Could you check a few things on this model? Use its own coordinates, in mm. Round coordinates to 2 decimals unless told otherwise and drop trailing zeros. Loops run counter-clockwise (first coordinate to the right, second up) from the corner with the lowest first, then second, coordinate; pieces in that order, holes last. Notation, with made-up numbers: M 72,27.5 L 80,27.5 A18 cw 80,33.5 Z; hole C -4,79 d3. An arc over 180 degrees is marked long. Answer in a Markdown table with one row per item.
Autodesk Inventor part; units mm, degrees
ref_plane "YZ Plane" through (0, 0, 0) normal (1, 0, 0) x (0, 1, 0)
ref_plane "XZ Plane" through (0, 0, 0) normal (0, 1, 0) x (-1, 0, 0)
ref_plane "XY Plane" through (0, 0, 0) normal (0, 0, 1) x (1, 0, 0)
ref_plane "Work Plane1" through (-228.0882, -76.2, -228.6) normal (0, 1, 0) x (-1, 0, 0)
sketch "Sketch2" plane through (-228.0882, -76.2, -228.6) normal (0, 1, 0) x (-1, 0, 0)
  circle A0 centre (-228.6, 228.6) radius 227.5764 construction
  circle A1 centre (-228.6, 228.6) radius 228.6 construction
  arc A2 (-228.6, 1.0236) -> (-25.4, 126.1267) centre (-228.6, 228.6) ccw construction
  arc A3 (-228.6, 0) -> (-25.4, 123.8731) centre (-228.6, 228.6) ccw construction
  line L0 (-228.6, 0) -> (-25.4, 0)
  arc A4 (-228.6, 1.0236) -> (-25.4, 126.1267) centre (-228.6, 228.6) ccw
  line L1 (-228.6, 228.6) -> (-25.4, 126.1267) construction
  line L2 (-228.6, 228.6) -> (-228.6, 1.0236) construction
  line L3 (-25.4, 126.1267) -> (-25.4, 0)
  line L4 (-228.6, 0) -> (-228.6, 1.0236)
  line L5 (-228.6, 0) -> (-228.6, 1.0236)
  line L6 (-25.4, 123.8731) -> (-25.4, 126.1267)
  point P0 (-228.0882, 228.6)
  point P1 (-1.0236, 228.6)
  point P2 (0, 228.6)
  point P3 (-228.6, 228.6)
  point P4 (-228.6, 228.6)
  dimension "d14" = 203.2
extrude "Extrusion1" add sketch "Sketch2" against normal blind 6.35
properties part number "Cyclone Inlet"
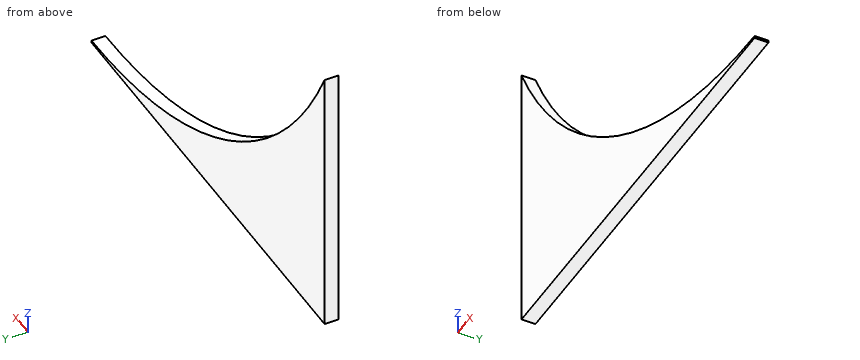
1) I want a section at A-A, the plane y = -79.25. Please give me the cut outline in (x, z), plus the area to 3 significant figures.
Computed:
| item | result |
|---|---|
| outline | M -202.69,-228.6 L 0.51,-228.6 L 0.51,-227.58 A227.58 cw -202.69,-102.47 Z |
| area | 7,460 mm² |
2) I want a section at B-B, the plane x = -124. Please give me the cut outline in (y, z).
Computed:
| item | result |
|---|---|
| outline | M -82.55,-228.6 L -76.2,-228.6 L -76.2,-190.49 L -82.55,-190.49 Z |
3) I need wall thicknesses on line 1 (Z direction, x = -161.5, y = -77.5); line 2 (Z direction, x = -108.5, y = -77.5); line 3 (X direction, y = -77.75, z = -202). Which ranges of each line are inside material? Lowest first, please.
Computed:
| item | result |
|---|---|
| line 1 | z = -228.6 to -159.82 |
| line 2 | z = -228.6 to -199.77 |
| line 3 | x = -202.69 to -104.31 |
4) Will these pins go through, and if not, where does the flat tip stop? P1, Ø1, axis at y = -79.5, z = -189.5, coming from the +X side; P2, Ø1, axis at y = -78.5, z = -166.5, coming from the +X side.
Computed:
| item | result |
|---|---|
| P1 | stops at x = -124.75 |
| P2 | stops at x = -154.09 |
